```python
from build123d import *

# Parameters (mm, degrees)
F0_W     = 80
F0_H     = 125
F1_DEPTH = 5
F3_D     = 6.6
F4_R     = 10


with BuildPart() as f1:
    # F0 (on Front) → F1 (new body)
    with BuildSketch(Plane.XZ):
        Rectangle(F0_W, F0_H)
    extrude(amount=F1_DEPTH)

    # F3 (through all)
    with Locations(Plane.XZ.offset(5)):
        with Locations((-25, -52.5), (25, -52.5)):
            Hole(F3_D / 2)

    # F4
    f4_edges = [f1.edges().sort_by_distance(p)[0] for p in [
        (40, -2.5, -62.5),
        (-40, -2.5, -62.5),
    ]]
    fillet(f4_edges, radius=F4_R)


solid = f1.part
```
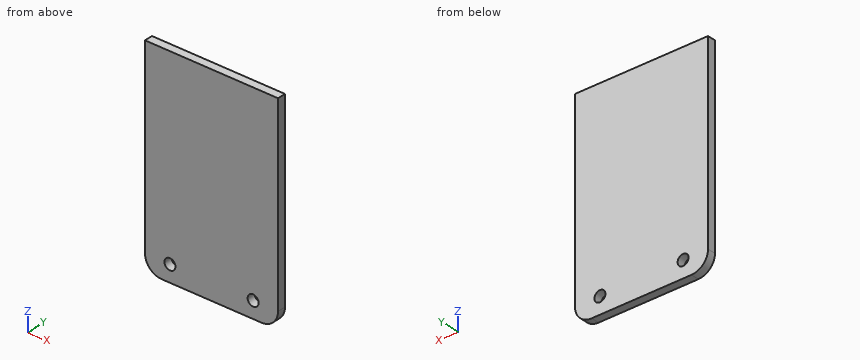
Read the model definition and answer for the solid it produces. Units are mm, in the model's axes. Coordinates: 2 decimals unless noted, no trailing zeros. Write each loop counter-clockwise with the first axis right and the second up, starting at its lowest first coordinate (ties: lowest second). Pieces come first, ordered by that corner, then holes. Notation, with made-up numbers: (-4.75, -35) -> (47.25, -35) arc R32 ccw to (47.25, -9) -> close; hole circle Ø7 at (69.5, 46.25). An arc over 180 degrees is marked (long way). Answer as a JSON object with one key per item and string values.
Q1. The part is cut by section A-A on x = -25. Give the vertices of the cut face in (y, z).
The answers:
{"outline": "(-5, -62.5) -> (0, -62.5) -> (0, -55.8) -> (-5, -55.8) -> close; (-5, -49.2) -> (0, -49.2) -> (0, 62.5) -> (-5, 62.5) -> close"}
Q2. The part is cut by section C-C on x = 26. Give the vertices of the cut face in (y, z).
The answers:
{"outline": "(-5, -62.5) -> (0, -62.5) -> (0, -55.64) -> (-5, -55.64) -> close; (-5, -49.36) -> (0, -49.36) -> (0, 62.5) -> (-5, 62.5) -> close"}
Q3. The part is cut by section B-B on z = -54.5. Give the vertices of the cut face in (x, y), then the cut area to 3 significant figures.
The answers:
{"outline": "(-39.8, -5) -> (-27.62, -5) -> (-27.62, 0) -> (-39.8, 0) -> close; (-22.38, -5) -> (22.38, -5) -> (22.38, 0) -> (-22.38, 0) -> close; (27.62, -5) -> (39.8, -5) -> (39.8, 0) -> (27.62, 0) -> close", "area": "345 mm2"}
Q4. Consider line 1 (Z direction, x = -25, y = -0.95); line 2 (X direction, y = -1.3, z = -51.5); line 3 (Z direction, x = -30.5, y = -1). Determine where each line is inside the solid, lowest interval first. Write a range as [from, to].
The answers:
{"line 1": "z = [-62.5, -55.8], [-49.2, 62.5]", "line 2": "x = [-40, -28.14], [-21.86, 21.86], [28.14, 40]", "line 3": "z = [-62.49, 62.5]"}
